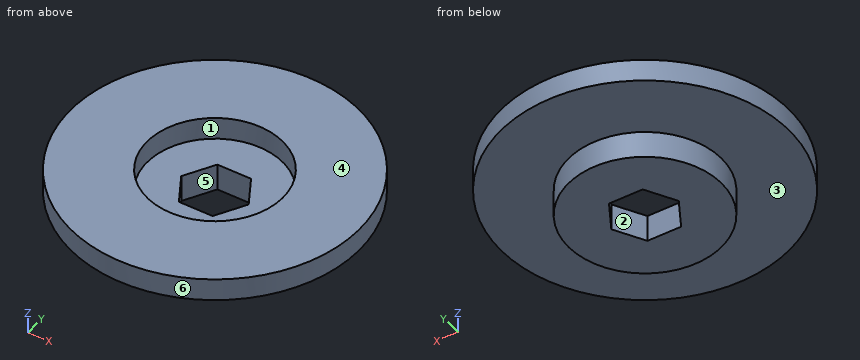
from build123d import *

# Parameters (mm, degrees)
EXTRUDE008_DEPTH = 10
SKETCH010_R      = 17
EXTRUDE007_DEPTH = 6
SKETCH008_R      = 32
SKETCH008_R_2    = 15.05
EXTRUDE006_DEPTH = 5


with BuildPart() as extrude008:
    # Sketch012 (on Face1 of CopyExtrude007001) → Extrude008 (new body)
    with BuildSketch(Plane(origin=(0, 0, -11), x_dir=(1, 0, 0), z_dir=(0, 0, -1))):
        Polygon((-3.752777, -6.5), (3.752777, -6.5), (7.505553, 0), (3.752777, 6.5), (-3.752777, 6.5), (-7.505553, 0), align=None)
    extrude(amount=-EXTRUDE008_DEPTH)


with BuildPart() as cut005:
    # Sketch010 (on Face1 of CopyExtrude006001) → Extrude007 (new body)
    with BuildSketch(Plane(origin=(0, 0, -5), x_dir=(1, 0, 0), z_dir=(0, 0, -1))):
        Circle(SKETCH010_R)
    extrude(amount=EXTRUDE007_DEPTH)

    # Cut005: cut Extrude008
    add(extrude008.part, mode=Mode.SUBTRACT)


with BuildPart() as fusion002:
    # Sketch008 (on Face1 of CopyCut004001) → Extrude006 (new body)
    with BuildSketch(Plane(origin=(0, 0, 0), x_dir=(1, 0, 0), z_dir=(0, 0, -1))):
        Circle(SKETCH008_R)
        Circle(SKETCH008_R_2, mode=Mode.SUBTRACT)
    extrude(amount=EXTRUDE006_DEPTH)

    # Fusion002: union Cut005
    add(cut005.part)


solid = fusion002.part
Input: part model. Units: mm. Frame: model coordinates. Face numbers are marked on the shaded views. A direction names the side the tool comes from. Round coordinates to 2 decimals unless told otherwise and drop trailing zeros. Loops run counter-clockwise (first coordinate to the right, second up) from the corner with the lowest first, then second, coordinate; pieces in that order, holes last. Notation, with made-up numbers: (84, 70) -> (99, 70) arc R17 cw to (99, 85) -> close; hole circle Ø11 at (25, -14). An arc over 180 degrees is marked (long way). Answer as a JSON object with one key per item and string values. Group by question number.
1) Section query A-A on x = 0. Output: boundary loops of the cut face in (y, z).
2) Section query D-D on y = 12.5. Output: boundary loops of the cut face in (x, z), plus the area to 3 significant figures.
3) Draft query along Y for the marked faces 4, 5 and 6. Return one class per face: +Y half, -Y half, draft (parallel to the pull), parting line (faces both ways), or undercut.
4) Section query C-C on y = 1. Output: boundary loops of the cut face in (x, z), plus the area to 3 significant figures.
5) Pin query (flat end, axial travel): pin 1 (3 mm diameter, centred on x = -21, y = 7, fed in from -Z); pin 2 (4 mm diameter, centred on x = 20, y = -15, fed in from +Z); pin 3 (4 mm diameter, centred on x = 24, z = -3, fed in from +Y); pin 4 (3 mm diameter, centred on y = -19, z = -6, fed in from +X). Return the tip coordinate at first contact, or that it passes through.
6) Section query B-B on z = -7.75. Output: boundary loops of the cut face in (x, y), plus the area to 3 significant figures.
7) Ray query, L1, parallel to Y at x = 0, z = -3.2; L2, parallel to Z at x = 9, y = -9.5. Return the intervals inside material, ascending.
8) Reachability of the marked faces 1, 2 and 3 from +Z, -Z, +X, -X, +Y, -Y: full face, straight path, thin tool, end or side. Return the list, or none.
Reply:
{
 "1": {"outline": "(-32, -5) -> (-17, -5) -> (-17, -11) -> (-6.5, -11) -> (-6.5, -5) -> (-15.05, -5) -> (-15.05, 0) -> (-32, 0) -> close; (6.5, -11) -> (17, -11) -> (17, -5) -> (32, -5) -> (32, 0) -> (15.05, 0) -> (15.05, -5) -> (6.5, -5) -> close"},
 "2": {"outline": "(-29.46, -5) -> (-11.52, -5) -> (-11.52, -11) -> (11.52, -11) -> (11.52, -5) -> (29.46, -5) -> (29.46, 0) -> (8.38, 0) -> (8.38, -5) -> (-8.38, -5) -> (-8.38, 0) -> (-29.46, 0) -> close", "area": "349 mm2"},
 "3": {"face 4": "draft", "face 5": "undercut", "face 6": "parting line"},
 "4": {"outline": "(-31.98, -5) -> (-16.97, -5) -> (-16.97, -11) -> (-6.93, -11) -> (-6.93, -5) -> (-15.02, -5) -> (-15.02, 0) -> (-31.98, 0) -> close; (6.93, -11) -> (16.97, -11) -> (16.97, -5) -> (31.98, -5) -> (31.98, 0) -> (15.02, 0) -> (15.02, -5) -> (6.93, -5) -> close", "area": "290 mm2"},
 "5": {"pin 1": "stops at z = -5", "pin 2": "stops at z = 0", "pin 3": "stops at y = 23.24", "pin 4": "stops at x = 26.54"},
 "6": {"outline": "circle Ø34 at (0, 0); hole (-7.51, 0) -> (-3.75, -6.5) -> (3.75, -6.5) -> (7.51, 0) -> (3.75, 6.5) -> (-3.75, 6.5) -> close", "area": "762 mm2"},
 "7": {"L1": "y = -32 to -15.05, 15.05 to 32", "L2": "z = -11 to -5"},
 "8": {"face 1": "+Z", "face 2": "+Z, -Z", "face 3": "-Z"}
}
